Here's how the part is built. I have some questions about the finished solid (model axes, mm). A direction names the side the tool comes from. Coordinates: 2 decimals unless noted, no trailing zeros. Loops run counter-clockwise (first coordinate to the right, second up) from the corner with the lowest first, then second, coordinate; pieces in that order, holes last. Notation, with made-up numbers: M -10,41.25 L 27,41.25 A30 cw 27,64.25 Z; hole C 50.5,-1.75 d9. An arc over 180 degrees is marked long. Use one line per item in the form item = value. Start each with the question number.
(1) Imagine slicing it at A-A, the plane x = 0. Please give me the cut outline in (y, z), and give its area (3 significant figures).
(2) Will these pins go through, and if not, where does the flat tip stop? P1, Ø0.5, axis at y = -0.5, z = 2.5, coming from the +X side; P2, Ø0.8, axis at x = 2, y = -0.5, coming from the +Z side; P3, Ø2.5, axis at x = 0.5, z = 7, coming from the -Y side.
(3) Please list where these lines run through material, in increasing order: L1, parallel to X at y = 0.3, z = 0.25; L2, parallel to Z at x = -5.75, y = -0.8; L3, parallel to Y at x = -8.25, z = 0.
(4) On a 3-axis mill with a long thin cutter (end or side, diameter ignored), from which of +Z, -Z, +X, -X, +Y, -Y can I reach the whole of each face in a straight line? I mean faces 1 (the cylindrical face through (-1.73, 1.49, 7.81)), 2 (the flat face through (-0.1, -0.5, -5)), 3 (the flat face through (-8.66, -0.5, -0.1)), 4 (the flat face through (8.66, -0.5, -0.1)). Say none if no direction works.
(5) Imagine slicing it at B-B, the plane z = 0. Please give me the cut outline in (x, y), and give its area (3 significant figures).
(6) Imagine slicing it at D-D, the plane z = 7.5. Please give me the cut outline in (x, y).
(7) Imagine slicing it at C-C, the plane y = -0.45. Please give me the cut outline in (x, z), and give its area (3 significant figures).
```python
from build123d import *

# Parameters (mm, degrees)
ESBO_O1_R                = 10
RESSALTO_EXTRUS_O1_DEPTH = 1
ESBO_O2_R                = 8
RESSALTO_EXTRUS_O2_DEPTH = 1
ESBO_O3_W                = 17.320508076
ESBO_O3_H                = 10
RESSALTO_EXTRUS_O3_DEPTH = 1


with BuildPart() as part:
    # Esboço1 → Ressalto-extrusão1 (new body)
    with BuildSketch(Plane(origin=(0, 0, 0), x_dir=(1, 0, 0), z_dir=(0, 1, 0))):
        Circle(ESBO_O1_R)
    extrude(amount=RESSALTO_EXTRUS_O1_DEPTH)

    # Esboço2 → Ressalto-extrusão2 (add)
    with BuildSketch(Plane(origin=(0, 1, 0), x_dir=(1, 0, 0), z_dir=(0, 1, 0))):
        Circle(ESBO_O2_R)
    extrude(amount=RESSALTO_EXTRUS_O2_DEPTH)

    # Esboço3 → Ressalto-extrusão3 (add)
    with BuildSketch(Plane.XZ):
        Rectangle(ESBO_O3_W, ESBO_O3_H)
    extrude(amount=RESSALTO_EXTRUS_O3_DEPTH)


solid = part.part
```
Answer:
q1.outline = M -1,-5 L 0,-5 L 0,-10 L 1,-10 L 1,-8 L 2,-8 L 2,8 L 1,8 L 1,10 L 0,10 L 0,5 L -1,5 Z
q1.area = 46.0 mm²
q2.P1 = 8.66
q2.P2 = 5
q2.P3 = 0
q3.L1 = -10 to 10
q3.L2 = -5 to 5
q3.L3 = -1 to 1
q4.face_1 = +Y
q4.face_2 = -Z, +X, -X, -Y
q4.face_3 = +Z, -Z, -X, -Y
q4.face_4 = +Z, -Z, +X, -Y
q5.outline = M -10,0 L -8.66,0 L -8.66,-1 L 8.66,-1 L 8.66,0 L 10,0 L 10,1 L 8,1 L 8,2 L -8,2 L -8,1 L -10,1 Z
q5.area = 53.3 mm²
q6.outline = M -6.61,0 L 6.61,0 L 6.61,1 L 2.78,1 L 2.78,2 L -2.78,2 L -2.78,1 L -6.61,1 Z
q7.outline = M -8.66,-5 L 8.66,-5 L 8.66,5 L -8.66,5 Z
q7.area = 173 mm²
